Design review of the part built by this model. Coordinates are the model's own, in mm. Round coordinates to 2 decimals unless told otherwise and drop trailing zeros. Order: outer loops, then holes, each group sorted by start corner. A loop starts at its lowest first (then second) coordinate and runs counter-clockwise, first axis right, second up.
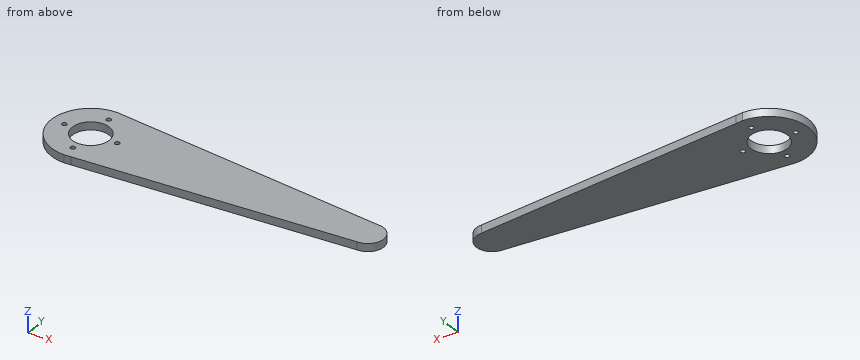
from build123d import *

# Parameters (mm, degrees)
SKETCH1_R           = 6
SKETCH1_R_2         = 0.9
SKETCH1_R_3         = 7
BOSS_EXTRUDE1_DEPTH = 3


with BuildPart() as part:
    # Sketch1 → Boss-Extrude1 (new body)
    # profile 1 of 3: a face of its own
    with BuildSketch(Plane.XY):
        with BuildLine():
            Line((105, 6), (2.55267423, 14.781199352))
            ThreePointArc((2.55267423, 14.781199352), (11.473667972, 9.662036187), (15, 0))
            ThreePointArc((15, 0), (11.473667972, -9.662036187), (2.55267423, -14.781199352))
            Line((2.55267423, -14.781199352), (105, -6))
            ThreePointArc((105, -6), (99, 0), (105, 6))
        make_face()
    # profile 2 of 3: a face of its own
    with BuildSketch(Plane.XY):
        with Locations((105, 0)):
            Circle(SKETCH1_R)
    # profile 3 of 3: a face of its own
    with BuildSketch(Plane.XY):
        with BuildLine():
            Line((2.55267423, 14.781199352), (0, 15))
            ThreePointArc((0, 15), (-15, 0), (0, -15))
            Line((0, -15), (2.55267423, -14.781199352))
            ThreePointArc((2.55267423, -14.781199352), (11.473667972, -9.662036187), (15, 0))
            ThreePointArc((15, 0), (11.473667972, 9.662036187), (2.55267423, 14.781199352))
        make_face()
        with Locations((0, -10)):
            Circle(SKETCH1_R_2, mode=Mode.SUBTRACT)
        with Locations((10, 0)):
            Circle(SKETCH1_R_2, mode=Mode.SUBTRACT)
        with Locations((-10, 0)):
            Circle(SKETCH1_R_2, mode=Mode.SUBTRACT)
        Circle(SKETCH1_R_3, mode=Mode.SUBTRACT)
        with Locations((0, 10)):
            Circle(SKETCH1_R_2, mode=Mode.SUBTRACT)
    extrude(amount=BOSS_EXTRUDE1_DEPTH)


solid = part.part
1) Take a section at C-C on x = 18. Give the boundary of the cut face in (y, z), plus the area to 3 significant figures.
Results:
outline: (-13.46, 0) - (13.46, 0) - (13.46, 3) - (-13.46, 3) - close
area: 80.7 mm2
2) Clearance check with a flat-ended pin moving along its axis: P1, Ø1, axis at x = 50.5, z = 0.5, coming from the -Y side. State where the tip first meets the part, or that it passes through.
Results:
P1: stops at y = -10.71
3) Take a section at A-A on z = 2.1. Give the boundary of the cut face in (x, y), plus the area to 3 significant figures.
Results:
outline: (0, -15) - (105, -6) arc R6 ccw to (105, 6) - (0, 15) arc R15 ccw to start; hole circle Ø1.8 at (-10, 0); hole circle Ø14 at (0, 0); hole circle Ø1.8 at (0, -10); hole circle Ø1.8 at (0, 10); hole circle Ø1.8 at (10, 0)
area: 2,450 mm2
4) Take a section at B-B on y = -2.5. Give the boundary of the cut face in (x, z).
Results:
outline: (-14.79, 0) - (-6.54, 0) - (-6.54, 3) - (-14.79, 3) - close; (6.54, 0) - (110.45, 0) - (110.45, 3) - (6.54, 3) - close
5) Take a section at D-D on x = 75. Give the boundary of the cut face in (y, z), plus the area to 3 significant figures.
Results:
outline: (-8.57, 0) - (8.57, 0) - (8.57, 3) - (-8.57, 3) - close
area: 51.4 mm2
6) To check wall thickness, follow line 1 along Y through (x, z) = (0, 2.25); line 2 along X through (y, z) = (2.25, 1.1); line 3 along Y through (x, z) = (-4, 1.8). State the ranges of each line that lie inside material, in increasing order.
Results:
line 1: y = -15 to -10.9, -9.1 to -7, 7 to 9.1, 10.9 to 15
line 2: x = -14.83 to -6.63, 6.63 to 110.56
line 3: y = -14.46 to -5.74, 5.74 to 14.46
